Work out the finished part from the listing and answer in its coordinate system (mm). A direction names the side the tool comes from. Round coordinates to 2 decimals unless told otherwise and drop trailing zeros. Write each loop counter-clockwise with the first axis right and the second up, starting at its lowest first coordinate (ties: lowest second). Pieces come first, ordered by that corner, then holes. Notation, with made-up numbers: M -18.75,70.25 L -6.75,70.25 A16 cw -6.75,77.25 Z; hole C 66,42 d2. An arc over 180 degrees is marked long. Answer in a Markdown table with one row per item.
```python
from build123d import *

# Parameters (mm, degrees)
SKETCH1_R           = 30
BOSS_EXTRUDE1_DEPTH = 3
SKETCH2_R           = 10
BOSS_EXTRUDE2_DEPTH = 6
SKETCH3_R           = 2.5
CUT_EXTRUDE1_DEPTH  = 44.370496884


with BuildPart() as part:
    # Sketch1 → Boss-Extrude1 (new body)
    with BuildSketch(Plane.XY):
        Circle(SKETCH1_R)
    extrude(amount=BOSS_EXTRUDE1_DEPTH)

    # Sketch2 → Boss-Extrude2 (add)
    with BuildSketch(Plane.XY.offset(3)):
        Circle(SKETCH2_R)
    extrude(amount=BOSS_EXTRUDE2_DEPTH)

    # Sketch3 → Cut-Extrude1 (cut, through all)
    with BuildSketch(Plane(origin=(0, 0, 0), x_dir=(-1, 0, 0), z_dir=(0, 0, -1))):
        with Locations((0, 25)):
            Circle(SKETCH3_R)
        with Locations((8.550503583, 23.49231552)):
            Circle(SKETCH3_R)
        with Locations((16.069690242, 19.151111078)):
            Circle(SKETCH3_R)
        with Locations((21.650635095, 12.5)):
            Circle(SKETCH3_R)
        with Locations((24.620193825, 4.341204442)):
            Circle(SKETCH3_R)
        with Locations((24.620193825, -4.341204442)):
            Circle(SKETCH3_R)
        with Locations((21.650635095, -12.5)):
            Circle(SKETCH3_R)
        with Locations((16.069690242, -19.151111078)):
            Circle(SKETCH3_R)
        with Locations((8.550503583, -23.49231552)):
            Circle(SKETCH3_R)
        with Locations((0, -25)):
            Circle(SKETCH3_R)
        with Locations((-8.550503583, -23.49231552)):
            Circle(SKETCH3_R)
        with Locations((-16.069690242, -19.151111078)):
            Circle(SKETCH3_R)
        with Locations((-21.650635095, -12.5)):
            Circle(SKETCH3_R)
        with Locations((-24.620193825, -4.341204442)):
            Circle(SKETCH3_R)
        with Locations((-24.620193825, 4.341204442)):
            Circle(SKETCH3_R)
        with Locations((-21.650635095, 12.5)):
            Circle(SKETCH3_R)
        with Locations((-16.069690242, 19.151111078)):
            Circle(SKETCH3_R)
        with Locations((-8.550503583, 23.49231552)):
            Circle(SKETCH3_R)
    extrude(amount=-CUT_EXTRUDE1_DEPTH, mode=Mode.SUBTRACT)


solid = part.part
```
1. The part is cut by section D-D (y = 25). Determine the outline of the cut face in (x, z).
Calculated:
| item | result |
|---|---|
| outline | M -16.58,0 L -10.54,0 L -10.54,3 L -16.58,3 Z; M -6.56,0 L -2.5,0 L -2.5,3 L -6.56,3 Z; M 2.5,0 L 6.56,0 L 6.56,3 L 2.5,3 Z; M 10.54,0 L 16.58,0 L 16.58,3 L 10.54,3 Z |
2. A tool of negligible diameter and unlimited length cuts with its end or side. For faces 1 (the cylindrical face through (7.21, -21.38, 1.48)), 2 (the cylindrical face through (-2.17, -9.76, 5.96)), from which of +Z, -Z, +X, -X, +Y, -Y can it reach the whole face along a straight path? Write none if from no direction.
Calculated:
| item | result |
|---|---|
| face 1 | +Z, -Z |
| face 2 | +Z |
3. The part is cut by section C-C (z = 2). Count the separate pieces of the cut face and the enclosed holes in it, plus the area to 3 significant figures.
Calculated:
| item | result |
|---|---|
| separate pieces | 1 |
| enclosed holes | 18 |
| area | 2,470 mm² |
4. Consider line 1 along X through (y, z) = (23.5, 1.5); line 2 along Z through (x, y) = (-16.5, 5.5); line 3 along X through (y, z) = (-24, 0.75). Determine where each line is inside the solid, lowest interval first. Write a range as from..to.
Calculated:
| item | result |
|---|---|
| line 1 | x = -18.65..-11.05, -6.05..-2, 2..6.05, 11.05..18.65 |
| line 2 | z = 0..3 |
| line 3 | x = -18..-11, -6.1..-2.29, 2.29..6.1, 11..18 |
5. The part is cut by section B-B (y = 12.5). Determine the outline of the cut face in (x, z).
Calculated:
| item | result |
|---|---|
| outline | M -27.27,0 L -24.15,0 L -24.15,3 L -27.27,3 Z; M -19.15,0 L 19.15,0 L 19.15,3 L -19.15,3 Z; M 24.15,0 L 27.27,0 L 27.27,3 L 24.15,3 Z |
6. Given pin 1 (4 mm diameter, centred on x = -7, y = -15.5, fed in from +Z), flat-ended and moving along its own axis, determine where the tip first touches the part or whether it passes through.
Calculated:
| item | result |
|---|---|
| pin 1 | stops at z = 3 |
7. The part is cut by section A-A (x = 0). Determine the outline of the cut face in (y, z).
Calculated:
| item | result |
|---|---|
| outline | M -30,0 L -27.5,0 L -27.5,3 L -30,3 Z; M -22.5,0 L 22.5,0 L 22.5,3 L 10,3 L 10,9 L -10,9 L -10,3 L -22.5,3 Z; M 27.5,0 L 30,0 L 30,3 L 27.5,3 Z |
8. Determine the mould class of faces 3 (the flat face through (13, 0, 3)), 4 (the cylindrical face through (-29.97, 1.32, 1.48)), 5 (the cylindrical face through (7.207, 25.6, 1.479)) for opening direction Y: released by +Y, released by -Y, zero draft, split by the parting line, or undercut.
Calculated:
| item | result |
|---|---|
| face 3 | zero draft |
| face 4 | split by the parting line |
| face 5 | undercut |
